from build123d import *

# Parameters (mm, degrees)
SKETCH1_R           = 2
SKETCH1_R_2         = 0.5
BOSS_EXTRUDE1_DEPTH = 2
BOSS_EXTRUDE2_START = 2
SKETCH1_3_R         = 2
BOSS_EXTRUDE2_DEPTH = 26


with BuildPart() as part:
    # Sketch1 → Boss-Extrude1 (new body)
    with BuildSketch(Plane(origin=(0, 0, 0), x_dir=(1, 0, 0), z_dir=(0, 1, 0))):
        with BuildLine():
            Line((2, 7.5), (2, 2.88735269))
            Line((2, 2.88735269), (17.117647059, 1.996536794))
            ThreePointArc((17.117647059, 1.996536794), (19, 0), (17.117647059, -1.996536794))
            Line((17.117647059, -1.996536794), (2, -2.88735269))
            Line((2, -2.88735269), (2, -7.5))
            ThreePointArc((2, -7.5), (0, -9.5), (-2, -7.5))
            Line((-2, -7.5), (-2, -2.88735269))
            Line((-2, -2.88735269), (-17.117647059, -1.996536794))
            ThreePointArc((-17.117647059, -1.996536794), (-19, 0), (-17.117647059, 1.996536794))
            Line((-17.117647059, 1.996536794), (-2, 2.88735269))
            Line((-2, 2.88735269), (-2, 7.5))
            ThreePointArc((-2, 7.5), (0, 9.5), (2, 7.5))
        make_face()
        Circle(SKETCH1_R, mode=Mode.SUBTRACT)
        with Locations((-17, 0)):
            Circle(SKETCH1_R_2, mode=Mode.SUBTRACT)
        with Locations((17, 0)):
            Circle(SKETCH1_R_2, mode=Mode.SUBTRACT)
        with Locations((-14.5, 0)):
            Circle(SKETCH1_R_2, mode=Mode.SUBTRACT)
        with Locations((-12, 0)):
            Circle(SKETCH1_R_2, mode=Mode.SUBTRACT)
        with Locations((-9.5, 0)):
            Circle(SKETCH1_R_2, mode=Mode.SUBTRACT)
        with Locations((-7, 0)):
            Circle(SKETCH1_R_2, mode=Mode.SUBTRACT)
        with Locations((-4.5, 0)):
            Circle(SKETCH1_R_2, mode=Mode.SUBTRACT)
        with Locations((4.5, 0)):
            Circle(SKETCH1_R_2, mode=Mode.SUBTRACT)
        with Locations((7, 0)):
            Circle(SKETCH1_R_2, mode=Mode.SUBTRACT)
        with Locations((9.5, 0)):
            Circle(SKETCH1_R_2, mode=Mode.SUBTRACT)
        with Locations((12, 0)):
            Circle(SKETCH1_R_2, mode=Mode.SUBTRACT)
        with Locations((14.5, 0)):
            Circle(SKETCH1_R_2, mode=Mode.SUBTRACT)
        with Locations((0, 7.5)):
            Circle(SKETCH1_R_2, mode=Mode.SUBTRACT)
        with Locations((0, 4.5)):
            Circle(SKETCH1_R_2, mode=Mode.SUBTRACT)
        with Locations((0, -4.5)):
            Circle(SKETCH1_R_2, mode=Mode.SUBTRACT)
        with Locations((0, -7.5)):
            Circle(SKETCH1_R_2, mode=Mode.SUBTRACT)
    extrude(amount=BOSS_EXTRUDE1_DEPTH)

    # Sketch1_3 → Boss-Extrude2 (add)
    with BuildSketch(Plane(origin=(0, 0, 0), x_dir=(1, 0, 0), z_dir=(0, 1, 0)).offset(BOSS_EXTRUDE2_START)):
        Circle(SKETCH1_3_R)
    extrude(amount=-BOSS_EXTRUDE2_DEPTH)


solid = part.part
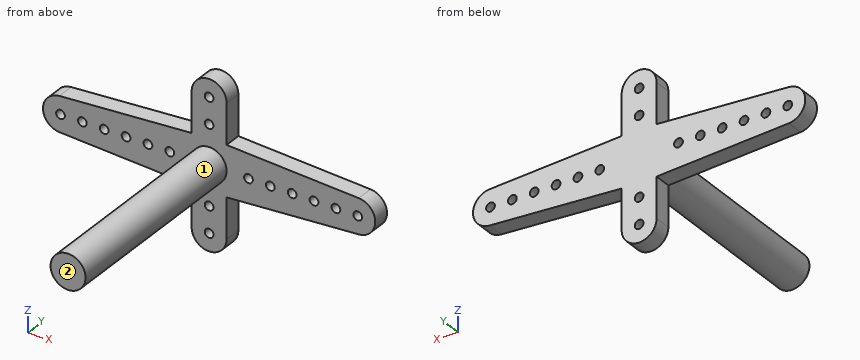
Build history of the part. All positions in model axes, mm. Face numbers are marked on the shaded views. A direction names the side the tool comes from. Round coordinates to 2 decimals unless told otherwise and drop trailing zeros. Write each loop counter-clockwise with the first axis right and the second up, starting at its lowest first coordinate (ties: lowest second). Pieces come first, ordered by that corner, then holes. Notation, with made-up numbers: M 52,86 L 68,86 A16 cw 68,117 Z; hole C 1.5,39.5 d11. An arc over 180 degrees is marked long. Answer as a JSON object with one key per item and string values. Group by question number.
(1) Which spindle directions (+Z, -Z, +X, -X, +Y, -Y) get a long thin tool onto all of the face, cutting with end or side? Do the marked faces 1 and 2. Say none if no direction does.
(2) Cut at C-C (z = -1). Give the cut face in (x, y).
(3) Cut at D-D (y = -13). Give the cut face in (x, z).
(4) Cut at A-A (x = 0). Give the cut face in (y, z), and give its area (3 significant figures).
(5) Drill centre lines: L1, parallel to X at y = 0.55, z = -7.5; L2, parallel to Z at x = -9.5, y = 0.85; L3, parallel to Y at x = 1, z = -8. Where is each one in solid material? Low to high.
(6) Cut at B-B (x = -12). Give the cut face in (y, z).
(7) Flat gauge pins, fed straight in: pin 1 (0.6 mm diameter, centred on y = 1.5, z = 5, fed in from +X); pin 2 (5 mm diameter, centred on x = -2, y = -17, fed in from +Z); pin 3 (1 mm diameter, centred on y = 1, z = 6.5, fed in from -X). Where does each tip first touch, or does it go through?
Responses:
{
 "1": {"face 1": "-Y", "face 2": "+Z, -Z, +X, -X, -Y"},
 "2": {"outline": "M -18.73,0 L -1.73,0 L -1.73,-24 L 1.73,-24 L 1.73,0 L 18.73,0 L 18.73,2 L -18.73,2 Z"},
 "3": {"outline": "C 0,0 d4"},
 "4": {"outline": "M -24,-2 L 0,-2 L 0,-4 L 2,-4 L 2,4 L 0,4 L 0,2 L -24,2 Z; M 0,-9.5 L 2,-9.5 L 2,-8 L 0,-8 Z; M 0,-7 L 2,-7 L 2,-5 L 0,-5 Z; M 0,5 L 2,5 L 2,7 L 0,7 Z; M 0,8 L 2,8 L 2,9.5 L 0,9.5 Z", "area": "126 mm2"},
 "5": {"L1": "x = -2 to -0.5, 0.5 to 2", "L2": "z = -2.45 to -0.5, 0.5 to 2.45", "L3": "y = 0 to 2"},
 "6": {"outline": "M 0,-2.3 L 2,-2.3 L 2,-0.5 L 0,-0.5 Z; M 0,0.5 L 2,0.5 L 2,2.3 L 0,2.3 Z"},
 "7": {"pin 1": "stops at x = 2", "pin 2": "stops at z = 2", "pin 3": "stops at x = -2"}
}
